```python
from build123d import *

# Parameters (mm, degrees)
SKETCH2_R                 = 11
BOSS_EXTRUDE2_DEPTH       = 25.4
SKETCH7_R                 = 4
CUT_EXTRUDE3_DEPTH        = 26.4
SKETCH8_R                 = 25.4
BOSS_EXTRUDE3_DEPTH       = 12.7
SKETCH10_R                = 4
CUT_EXTRUDE5_DEPTH        = 13.7
F_1_4_20_TAPPED_HOLE1_D   = 5.1054
M4X0_7_TAPPED_HOLE2_D     = 3.3
M4X0_7_TAPPED_HOLE2_DEPTH = 11.176
M4X0_7_TAPPED_HOLE2_TIP   = 0.991420021


with BuildPart() as part:
    # Sketch2 → Boss-Extrude2 (new body)
    with BuildSketch(Plane(origin=(0, 0, 0), x_dir=(0, 0, -1), z_dir=(1, 0, 0))):
        Circle(SKETCH2_R)
    extrude(amount=BOSS_EXTRUDE2_DEPTH)

    # Sketch7 → Cut-Extrude3 (cut, through all)
    with BuildSketch(Plane(origin=(25.4, 0, 0), x_dir=(0, 0, -1), z_dir=(1, 0, 0))):
        Circle(SKETCH7_R)
    extrude(amount=-CUT_EXTRUDE3_DEPTH, mode=Mode.SUBTRACT)

    # Sketch8 → Boss-Extrude3 (add)
    with BuildSketch(Plane.ZY):
        Circle(SKETCH8_R)
    extrude(amount=BOSS_EXTRUDE3_DEPTH)

    # Sketch10 → Cut-Extrude5 (cut, through all)
    with BuildSketch(Plane(origin=(0, 0, 0), x_dir=(0, 0, -1), z_dir=(1, 0, 0))):
        Circle(SKETCH10_R)
    extrude(amount=-CUT_EXTRUDE5_DEPTH, mode=Mode.SUBTRACT)

    # 1/4-20 Tapped Hole1 (through all)
    with Locations(Plane(origin=(-4.921208149, 25.4, 0), x_dir=(0, 0, 1), z_dir=(0, 1, 0))):
        with Locations((0, 0)):
            Hole(F_1_4_20_TAPPED_HOLE1_D / 2)

    # M4x0.7 Tapped Hole2
    with Locations(Plane(origin=(2.900798662, 11, 0), x_dir=(0, 0, 1), z_dir=(0, 1, 0))):
        with Locations((0, 0)):
            Hole(M4X0_7_TAPPED_HOLE2_D / 2, depth=M4X0_7_TAPPED_HOLE2_DEPTH)
            with Locations((0, 0, -(M4X0_7_TAPPED_HOLE2_DEPTH + M4X0_7_TAPPED_HOLE2_TIP / 2))):  # 118° drill point
                Cone(0, M4X0_7_TAPPED_HOLE2_D / 2, M4X0_7_TAPPED_HOLE2_TIP, mode=Mode.SUBTRACT)


solid = part.part
```
Geometry: final body of the model. Coordinates: model frame, mm. A direction names the side the tool comes from. Coordinates: 2 decimals unless noted, no trailing zeros. Order: outer loops, then holes, each group sorted by start corner. A loop starts at its lowest first (then second) coordinate and runs counter-clockwise, first axis right, second up. Notation, with made-up numbers: (22, 61) -> (71, 61) arc R14 ccw to (71, 77) -> close; hole circle Ø3 at (-30, 63). An arc over 180 degrees is marked (long way). Answer in a Markdown table with one row per item.
Item 1: Section D-D on y = 10. Output: boundary loops of the cut face in (x, z).
Return value:
| item | result |
|---|---|
| outline | (-12.7, -23.35) -> (0, -23.35) -> (0, -4.58) -> (25.4, -4.58) -> (25.4, 4.58) -> (0, 4.58) -> (0, 23.35) -> (-12.7, 23.35) -> close; hole circle Ø5.11 at (-4.92, 0); hole circle Ø3.3 at (2.9, 0) |
Item 2: Draft query along Y for faces 3 (the cylindrical face through (4.537, 7.272, 0.215)), 4 (the cylindrical face through (6.617, -3.905, 0.867)), 5 (the cylindrical face through (-6.261, -24.796, -5.506)). Return one class per face: released by +Y, released by -Y, zero draft, split by the parting line, or undercut.
Return value:
| item | result |
|---|---|
| face 3 | zero draft |
| face 4 | undercut |
| face 5 | split by the parting line |
Item 3: Section B-B on z = 0. Output: boundary loops of the cut face in (x, y), plus the area to 3 significant figures.
Return value:
| item | result |
|---|---|
| outline | (-12.7, -25.4) -> (-7.47, -25.4) -> (-7.47, -4) -> (-12.7, -4) -> close; (-12.7, 4) -> (-7.47, 4) -> (-7.47, 25.4) -> (-12.7, 25.4) -> close; (-2.37, -25.4) -> (0, -25.4) -> (0, -11) -> (25.4, -11) -> (25.4, -4) -> (-2.37, -4) -> close; (-2.37, 4) -> (1.25, 4) -> (1.25, 11) -> (0, 11) -> (0, 25.4) -> (-2.37, 25.4) -> close; (4.55, 4) -> (25.4, 4) -> (25.4, 11) -> (4.55, 11) -> close |
| area | 658 mm² |
Item 4: Ray query, L1, parallel to X at y = 6, z = 0; L2, parallel to X at y = 13, z = 9.5; L3, parallel to X at y = -12.25, z = 0. Return the intervals inside material, ascending.
Return value:
| item | result |
|---|---|
| L1 | x = -12.7 to -7.47, -2.37 to 1.25, 4.55 to 25.4 |
| L2 | x = -12.7 to 0 |
| L3 | x = -12.7 to -7.47, -2.37 to 0 |
Item 5: Section C-C on x = -6. Output: boundary loops of the cut face in (y, z).
Return value:
| item | result |
|---|---|
| outline | (-25.29, -2.31) arc R25.4 ccw to (25.29, -2.31) -> (3.26, -2.31) arc R4 cw to (-3.26, -2.31) -> close; (-25.29, 2.31) -> (-3.26, 2.31) arc R4 cw to (3.26, 2.31) -> (25.29, 2.31) arc R25.4 ccw to start |
Item 6: Section A-A on y = 0. Output: boundary loops of the cut face in (x, z).
Return value:
| item | result |
|---|---|
| outline | (-12.7, -25.4) -> (0, -25.4) -> (0, -11) -> (25.4, -11) -> (25.4, -4) -> (-12.7, -4) -> close; (-12.7, 4) -> (25.4, 4) -> (25.4, 11) -> (0, 11) -> (0, 25.4) -> (-12.7, 25.4) -> close |
Item 7: Contact query for flat-ended pins moving along their axis: P1, Ø10, axis at y = 11, z = 5.5, coming from the +X side; P2, Ø6, axis at x = -2, y = -4, coming from the +Z side; P3, Ø8, axis at x = -4, y = -12.5, coming from the -Z side; P4, Ø3, axis at x = 2.9, z = 0, coming from the +Y side. Output: stop coordinate, or through.
Return value:
| item | result |
|---|---|
| P1 | stops at x = 25.4 |
| P2 | stops at z = 25.38 |
| P3 | stops at z = -23.94 |
| P4 | stops at y = -3.71 |
Item 8: Access query for faces 1 (the flat face through (0, -5, 11)), 2 (the flat face through (-12.7, 0, 5)). Directions: +Z, -Z, +X, -X, +Y, -Y. A direction counts if a zero-diameter tool reaches every point of the face in a straight line with its end or side. Return the directions, or none.
Return value:
| item | result |
|---|---|
| face 1 | +X |
| face 2 | +Z, -Z, -X, +Y, -Y |
